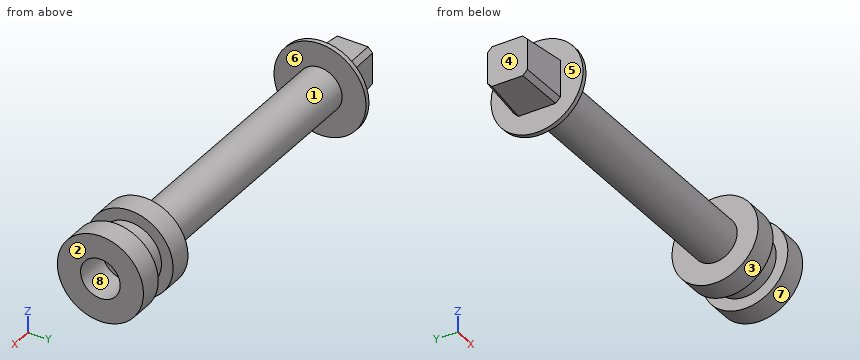
from build123d import *
from OCP.BRepFilletAPI import BRepFilletAPI_MakeChamfer

# Parameters (mm, degrees)
ESQUISSE2_W        = 40
ESQUISSE2_H        = 40
BOSS_EXTRU_1_DEPTH = 40
BOSS_EXTRU_1_TAPER = 4
CHANFREIN1_SIZE    = 4
CHANFREIN1_SIZE2   = 4.019606856


with BuildPart() as part:
    # Esquisse1 → Révolution1 (revolve)
    with BuildSketch(Plane.XY, mode=Mode.PRIVATE) as r_volution1_sk:
        Polygon((0, 0), (0, 39.5), (4, 39.5), (4, 19), (240, 19), (240, 37), (260, 37), (260, 27), (280, 27), (280, 37), (300, 37), (300, 17), (270, 17), (270, 0), align=None)
    revolve(r_volution1_sk.sketch.rotate(Axis((0, 0, 0), (1, 0, 0)), 90), axis=Axis((0, 0, 0), (1, 0, 0)))

    # Esquisse2 → Boss.-Extru.1 (add)
    with BuildSketch(Plane.ZY):
        Rectangle(ESQUISSE2_W, ESQUISSE2_H)
    extrude(amount=BOSS_EXTRU_1_DEPTH, taper=BOSS_EXTRU_1_TAPER)

    # Chanfrein1: one chamfer whose edges measure the first distance from different faces: ONE call of the kernel's chamfer builder (chamfer() names one face for all edges)
    chanfrein1_edges_1 = [part.edges().sort_by_distance(p)[0] for p in [
        (-20, 18.601463761, -18.601463761),
    ]]
    chanfrein1_side_1 = [part.faces().sort_by_distance(p)[0] for p in [
        (-19.498771976, 18.636513039, 0),
    ]]
    chanfrein1_edges_2 = [part.edges().sort_by_distance(p)[0] for p in [
        (-20, -18.601463761, -18.601463761),
    ]]
    chanfrein1_side_2 = [part.faces().sort_by_distance(p)[0] for p in [
        (-19.498771976, 0, -18.636513039),
    ]]
    chanfrein1_edges_3 = [part.edges().sort_by_distance(p)[0] for p in [
        (-20, -18.601463761, 18.601463761),
    ]]
    chanfrein1_side_3 = [part.faces().sort_by_distance(p)[0] for p in [
        (-19.498771976, -18.636513039, 0),
    ]]
    chanfrein1_edges_4 = [part.edges().sort_by_distance(p)[0] for p in [
        (-20, 18.601463761, 18.601463761),
    ]]
    chanfrein1_side_4 = [part.faces().sort_by_distance(p)[0] for p in [
        (-19.498771976, 0, 18.636513039),
    ]]
    chanfrein1 = BRepFilletAPI_MakeChamfer(part.part.solid().wrapped)
    for e in chanfrein1_edges_1:
        chanfrein1.Add(CHANFREIN1_SIZE, CHANFREIN1_SIZE2, e.wrapped, chanfrein1_side_1[0].wrapped)  # the first distance lies on this face
    for e in chanfrein1_edges_2:
        chanfrein1.Add(CHANFREIN1_SIZE, CHANFREIN1_SIZE2, e.wrapped, chanfrein1_side_2[0].wrapped)  # the first distance lies on this face
    for e in chanfrein1_edges_3:
        chanfrein1.Add(CHANFREIN1_SIZE, CHANFREIN1_SIZE2, e.wrapped, chanfrein1_side_3[0].wrapped)  # the first distance lies on this face
    for e in chanfrein1_edges_4:
        chanfrein1.Add(CHANFREIN1_SIZE, CHANFREIN1_SIZE2, e.wrapped, chanfrein1_side_4[0].wrapped)  # the first distance lies on this face
    add(Compound.cast(chanfrein1.Shape()), mode=Mode.REPLACE)


solid = part.part
CAD build for the part. Positions are in the model's coordinates, mm. Face numbers are marked on the shaded views. A direction names the side the tool comes from. Give positions to 0.01 mm unless a question says otherwise; leave off trailing zeros. Loops run counter-clockwise (first coordinate to the right, second up) from the corner with the lowest first, then second, coordinate; pieces in that order, holes last. Notation, with made-up numbers: M 0,81 L 29,81 A30 ccw 29,115 Z; hole C -11.5,-35 d6. An arc over 180 degrees is marked long. Write each question's results on one line, items separated by ' | '.
Q1. Flat gauge pins, fed straight in: P1, Ø10, axis at x = 207, y = 0.5, coming from the +Z side; P2, Ø8, axis at y = 31, z = -8.5, coming from the -X side; P3, Ø1, axis at x = 151, y = 14, coming from the +Z side. Where does each tip first touch, or does it go through?
Geometry check:
P1: stops at z = 19 | P2: stops at x = 0 | P3: stops at z = 13.37
Q2. Which spindle directions (+Z, -Z, +X, -X, +Y, -Y) get a long thin tool onto all of the face, cutting with end or side? Do the marked faces 1, 2, 3, 4 and 5. Say none if no direction does.
Geometry check:
face 1: none | face 2: +Z, -Z, +X, +Y, -Y | face 3: +X | face 4: +Z, -Z, -X, +Y, -Y | face 5: -X
Q3. Band-saw the part on B-B on z = 30. Write the cut outline in (x, y).
Geometry check:
outline: M 0,-25.7 L 4,-25.7 L 4,25.7 L 0,25.7 Z; M 240,-21.66 L 260,-21.66 L 260,21.66 L 240,21.66 Z; M 280,-21.66 L 300,-21.66 L 300,21.66 L 280,21.66 Z
Q4. Mould opens along Z. For the marked faces 6, 7 and 8 say: pulls with the +Z half, pulls with the -Z half, needs draft (parallel to the pull), parting line crosses it, or undercut.
Geometry check:
face 6: needs draft | face 7: parting line crosses it | face 8: undercut
Q5. Band-saw the part on A-A on y = -31. Write the cut outline in (x, z), and give its area (3 significant figures).
Geometry check:
outline: M 0,-24.48 L 4,-24.48 L 4,24.48 L 0,24.48 Z; M 240,-20.2 L 260,-20.2 L 260,20.2 L 240,20.2 Z; M 280,-20.2 L 300,-20.2 L 300,20.2 L 280,20.2 Z | area: 1,810 mm²
Q6. Probe probe 1 along X at (y, z) = (11, -34.5); probe 2 along Y at (x, z) = (280.5, 0); probe 3 along Y at (x, z) = (277, 0). List the from-to ranges inside material, lowest first.
Geometry check:
probe 1: x = 0 to 4, 240 to 260, 280 to 300 | probe 2: y = -37 to -17, 17 to 37 | probe 3: y = -27 to -17, 17 to 27
Q7. Band-saw the part on C-C on x = 224.5. Write the cut outline in (y, z).
Geometry check:
outline: C 0,0 d38
